from build123d import *

# Parameters (mm, degrees)
EXTRUDE1_DEPTH     = 2.413
CUT_EXTRUDE1_REACH = 4.413
SKETCH4_R          = 3.175


with BuildPart() as part:
    # Sketch1 → Extrude1 (new body)
    with BuildSketch(Plane.XY):
        with BuildLine():
            Line((111.27866266, 131.559165896), (125.42646266, 131.559165896))
            ThreePointArc((125.42646266, 131.559165896), (131.05256266, 125.933065896), (125.42646266, 120.306965896))
            Line((125.42646266, 120.306965896), (111.27866266, 120.306965896))
            ThreePointArc((111.27866266, 120.306965896), (105.65256266, 125.933065896), (111.27866266, 131.559165896))
        make_face()
    extrude(amount=EXTRUDE1_DEPTH)

    # Sketch4 → Cut-Extrude1 (cut, up to next)
    with BuildSketch(Plane.XY.offset(2.413), mode=Mode.PRIVATE) as cut_extrude1_sk1:
        with Locations((118.35256266, 125.933065896)):
            Circle(SKETCH4_R)
    cut_extrude1_tool1 = extrude(cut_extrude1_sk1.sketch, amount=-CUT_EXTRUDE1_REACH, mode=Mode.PRIVATE) & part.part
    add(cut_extrude1_tool1.solids().sort_by_distance((118.352563, 125.933066, 2.413))[0], mode=Mode.SUBTRACT)


solid = part.part
Design review of the part built by this model. Coordinates are the model's own, in mm. Coordinates: 2 decimals unless noted, no trailing zeros. Loops run counter-clockwise (first coordinate to the right, second up) from the corner with the lowest first, then second, coordinate; pieces in that order, holes last. Notation, with made-up numbers: M -16.5,12.25 L 34.5,12.25 A24 ccw 34.5,48.25 Z; hole C 66,40.5 d11. An arc over 180 degrees is marked long. Answer as CSV lines item,"result".
Item 1: For probe 1 along X at (y, z) = (125.75, 1.6); probe 2 along X at (y, z) = (124.5, 1.3); probe 3 along Y at (x, z) = (115.75, 1.6), list the stretches that pass through material, from the lowest coordinate up.
Answer list:
probe 1,"105.66 to 115.18, 121.52 to 131.05"
probe 2,"105.84 to 115.52, 121.19 to 130.87"
probe 3,"120.31 to 124.11, 127.75 to 131.56"
Item 2: Add section C-C on z = 0.9. State the section outline as (x, y) points (3 decimals), plus the area to 3 significant figures.
Answer list:
outline,"M 111.279,120.307 L 125.426,120.307 A5.626 ccw 125.426,131.559 L 111.279,131.559 A5.626 ccw Z; hole C 118.353,125.933 d6.35"
area,"227 mm²"
Item 3: The part is to be moulded in two halves that separate along X. For faces 1 (the face through (105.654, 125.809, 1.19)), 2 (the face through (121.4, 127.3, 0)), 3 (the face through (131.05, 126.06, 1.19)), 4 (the face through (115.833, 124.001, 1.223)), say which applies: pulls with the +X half, pulls with the -X half, needs draft (parallel to the pull), parting line crosses it, or undercut.
Answer list:
face 1,"pulls with the -X half"
face 2,"needs draft"
face 3,"pulls with the +X half"
face 4,"undercut"
Item 4: For P1, Ø1, axis at x = 109, z = 2, coming from the -Y side; P2, Ø1, axis at x = 127.5, y = 126.5, coming from the -Z side; P3, Ø1, axis at x = 127.5, z = 0.5, coming from the +Y side; P4, Ø5, axis at x = 118.35, y = 125.93, coming from the +Z side, all flat-tipped, find the tip position at first contact; note any pin that passes through.
Answer list:
P1,"y = 120.6"
P2,"z = 0"
P3,"y = 131.33"
P4,"through"
Item 5: Add section B-B on y = 124.25. State the section outline as (x, z) points, plus the area to 3 significant figures.
Answer list:
outline,"M 105.91,0 L 115.66,0 L 115.66,2.41 L 105.91,2.41 Z; M 121.04,0 L 130.79,0 L 130.79,2.41 L 121.04,2.41 Z"
area,"47.1 mm²"
Item 6: Add section D-D on y = 130.5. State the section outline as (x, z) points.
Answer list:
outline,"M 107.99,0 L 128.71,0 L 128.71,2.41 L 107.99,2.41 Z"
Item 7: Add section A-A on x = 115.75. State the section outline as (y, z) points, plus the area to 3 significant figures.
Answer list:
outline,"M 120.31,0 L 124.11,0 L 124.11,2.41 L 120.31,2.41 Z; M 127.75,0 L 131.56,0 L 131.56,2.41 L 127.75,2.41 Z"
area,"18.4 mm²"
